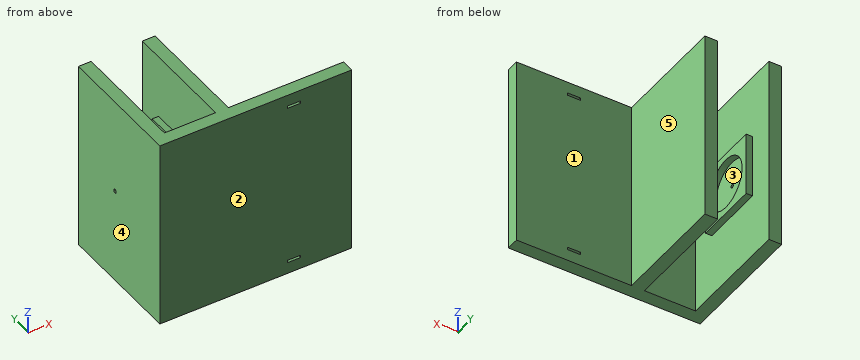
from build123d import *

# Parameters (mm, degrees)
BOSS_EXTRUDE1_DEPTH = 150
SKETCH3_W           = 10
SKETCH3_H           = 2
CUT_EXTRUDE1_DEPTH  = 10
SKETCH4_W           = 50
SKETCH4_H           = 50
SKETCH4_R           = 20
BOSS_EXTRUDE2_DEPTH = 5
BOSS_EXTRUDE3_START = 5
SKETCH5_W           = 50
SKETCH5_H           = 50
SKETCH5_R           = 20
BOSS_EXTRUDE3_DEPTH = 5
SKETCH6_R           = 1.5
CUT_EXTRUDE2_DEPTH  = 229.25424421


with BuildPart() as part:
    # Sketch1 → Boss-Extrude1 (new body)
    with BuildSketch(Plane.XY):
        Polygon((50, 100), (50, 10), (10, 10), (10, 100), (0, 100), (0, 10), (0, 0), (10, 0), (150, 0), (150, 10), (60, 10), (60, 100), align=None)
    extrude(amount=BOSS_EXTRUDE1_DEPTH)

    # Sketch3 → Cut-Extrude1 (cut)
    with BuildSketch(Plane(origin=(0, 10, 0), x_dir=(1, 0, 0), z_dir=(0, 1, 0))):
        with Locations((105, -10)):
            Rectangle(SKETCH3_W, SKETCH3_H)
        with Locations((105, -140)):
            Rectangle(SKETCH3_W, SKETCH3_H)
    extrude(amount=-CUT_EXTRUDE1_DEPTH, mode=Mode.SUBTRACT)

    # Sketch4 → Boss-Extrude2 (add)
    with BuildSketch(Plane(origin=(10, 0, 0), x_dir=(0, 0, -1), z_dir=(1, 0, 0))):
        with Locations((-75, 55)):
            Rectangle(SKETCH4_W, SKETCH4_H)
        with Locations((-75, 55)):
            Circle(SKETCH4_R, mode=Mode.SUBTRACT)
    extrude(amount=BOSS_EXTRUDE2_DEPTH)

    # Sketch5 → Boss-Extrude3 (add)
    with BuildSketch(Plane.ZY.offset(-50).offset(BOSS_EXTRUDE3_START)):
        with Locations((75, 55)):
            Rectangle(SKETCH5_W, SKETCH5_H)
        with Locations(Location((75, 55, 0), (0, 0, 180))):
            Circle(SKETCH5_R, mode=Mode.SUBTRACT)
    extrude(amount=-BOSS_EXTRUDE3_DEPTH)

    # Sketch6 → Cut-Extrude2 (cut, through all)
    with BuildSketch(Plane(origin=(10, 0, 0), x_dir=(0, 0, -1), z_dir=(1, 0, 0))):
        with Locations((-75, 55)):
            Circle(SKETCH6_R)
    extrude(amount=-CUT_EXTRUDE2_DEPTH, mode=Mode.SUBTRACT)


solid = part.part
Could you check a few things on this model? Use its own coordinates, in mm. Face numbers are marked on the shaded views. A direction names the side the tool comes from. Round coordinates to 2 decimals unless told otherwise and drop trailing zeros. Order: outer loops, then holes, each group sorted by start corner. A loop starts at its lowest first (then second) coordinate and runs counter-clockwise, first axis right, second up.
Q1. I'm going to push flat-ended pins straight in: P1, Ø5, axis at x = 31.5, z = 121.5, coming from the +Y side; P2, Ø4, axis at y = 75, z = 39, coming from the +X side. Where does each tip first touch, or does it pass through?
Geometry says:
P1: stops at y = 10
P2: stops at x = 60
Q2. Thinking about a two-plate mould opening in X: for the marked faces 3, 4 and 5, which applies, released by +X, released by -X, zero draft, split by the parting line, or undercut?
Geometry says:
face 3: undercut
face 4: released by -X
face 5: released by +X
Q3. Imagine slicing it at A-A, the plane y = 90.5. List the corners of the cut face in (x, z) for me.
Geometry says:
outline: (0, 0) - (10, 0) - (10, 150) - (0, 150) - close; (50, 0) - (60, 0) - (60, 150) - (50, 150) - close
Q4. Imagine slicing it at C-C, the plane z = 20. List the corners of the cut face in (x, y) for me, then the cut area to 3 significant figures.
Geometry says:
outline: (0, 0) - (150, 0) - (150, 10) - (60, 10) - (60, 100) - (50, 100) - (50, 10) - (10, 10) - (10, 100) - (0, 100) - close
area: 3,300 mm2
Q5. Imagine slicing it at B-B, the plane x = 102.5. List the corners of the cut face in (y, z) for me, then the cut area to 3 significant figures.
Geometry says:
outline: (0, 0) - (10, 0) - (10, 9) - (0, 9) - close; (0, 11) - (10, 11) - (10, 139) - (0, 139) - close; (0, 141) - (10, 141) - (10, 150) - (0, 150) - close
area: 1,460 mm2
Q6. Which directions (+Z, -Z, +X, -X, +Y, -Y) give clear straight access to the entire face, cutting with the end or side of a thin tool? Please do the marked faces 1 and 2.
Geometry says:
face 1: +Z, -Z, +X, +Y
face 2: +Z, -Z, +X, -X, -Y
Q7. Please list where these lines run through material, in increasing order: probe 1 along Y at (x, z) = (11.5, 76); probe 2 along Y at (x, z) = (4, 75); probe 3 along X at (y, z) = (62.5, 66.5).
Geometry says:
probe 1: y = 0 to 10, 30 to 35.03, 74.97 to 80
probe 2: y = 0 to 53.5, 56.5 to 100
probe 3: x = 0 to 10, 50 to 60
Q8. Imagine slicing it at D-D, the plane y = 47. List the corners of the cut face in (x, z) for me.
Geometry says:
outline: (0, 0) - (10, 0) - (10, 50) - (15, 50) - (15, 56.67) - (10, 56.67) - (10, 93.33) - (15, 93.33) - (15, 100) - (10, 100) - (10, 150) - (0, 150) - close; (45, 50) - (50, 50) - (50, 0) - (60, 0) - (60, 150) - (50, 150) - (50, 100) - (45, 100) - (45, 93.33) - (50, 93.33) - (50, 56.67) - (45, 56.67) - close
